from build123d import *

# Parameters (mm, degrees)
SKETCH1_R             = 52.3875
SKETCH1_R_2           = 27.49999999
BOSS_EXTRUDE1_DEPTH   = 11.43
M6_CLEARANCE_HOLE1_D  = 6.6
F_5_0MM_DOWEL_HOLE1_D = 5
CIRPATTERN1_COUNT     = 4
CUT_EXTRUDE1_DEPTH    = 284.979078357
CUT_EXTRUDE2_DEPTH    = 284.979078357


with BuildPart() as part:
    # Sketch1 → Boss-Extrude1 (new body)
    with BuildSketch(Plane(origin=(0, 0, 0), x_dir=(1, 0, 0), z_dir=(0, 1, 0))):
        with BuildLine():
            Line((-207.974881785, -9.956762437), (-62.780706514, -68.14502812))
            ThreePointArc((-62.780706514, -68.14502812), (-33.518744337, -68.231765471), (-12.176603989, -48.212200061))
            Line((-12.176603989, -48.212200061), (1.412558245, -19.284326264))
            ThreePointArc((1.412558245, -19.284326264), (9.075779399, -13.857488875), (17.670000792, -17.640990049))
            Line((17.670000792, -17.640990049), (83.271163186, -105.631794066))
            ThreePointArc((83.271163186, -105.631794066), (87.219797031, -141.651403947), (57.667100455, -162.619048791))
            Line((57.667100455, -162.619048791), (-117.895657849, -177.687193688))
            ThreePointArc((-117.895657849, -177.687193688), (-142.761859432, -174.739029029), (-164.426538493, -162.182702446))
            ThreePointArc((-164.426538493, -162.182702446), (-168.164823601, -160.06920649), (-172.443362527, -159.700770109))
            Line((-172.443362527, -159.700770109), (-204.355245166, -163.82191268))
            ThreePointArc((-204.355245166, -163.82191268), (-214.295764489, -158.206433226), (-211.707233022, -147.086764223))
            Line((-211.707233022, -147.086764223), (-198.151371623, -135.681934472))
            ThreePointArc((-198.151371623, -135.681934472), (-188.283833694, -119.954004575), (-189.430137427, -101.422354045))
            Line((-189.430137427, -101.422354045), (-220.388836369, -22.267635732))
            ThreePointArc((-220.388836369, -22.267635732), (-218.225236723, -12.034965467), (-207.974881785, -9.956762437))
        make_face()
        with Locations(Location((-123.19, -116.001477372, 0), (0, 0, 270))):
            Circle(SKETCH1_R, mode=Mode.SUBTRACT)
        with Locations(Location((54.61, -127, 0), (0, 0, 270))):
            Circle(SKETCH1_R_2, mode=Mode.SUBTRACT)
    extrude(amount=BOSS_EXTRUDE1_DEPTH)

    # M6 Clearance Hole1 (through all)
    with Locations(Plane(origin=(0, 0, 0), x_dir=(-1, 0, 0), z_dir=(0, -1, 0))):
        with Locations((-10.033704867, -23.334197365), (211.518182886, -18.798178744), (205.575185514, -154.375359311)):
            Hole(M6_CLEARANCE_HOLE1_D / 2)

    # Ø5.0mm Dowel Hole1 (through all)
    with Locations(Plane(origin=(0, 0, 0), x_dir=(-1, 0, 0), z_dir=(0, -1, 0))):
        with Locations((123.19, -173.151477372)):
            f_5_0mm_dowel_hole1 = Hole(F_5_0MM_DOWEL_HOLE1_D / 2)

    # CirPattern1: Ø5.0mm Dowel Hole1 ×4 about axis
    cirpattern1_axis = Axis((-123.19, 0, 116.001477372), (0, 1, 0))
    for i in range(1, CIRPATTERN1_COUNT):
        add(f_5_0mm_dowel_hole1.rotate(cirpattern1_axis, i * 360 / CIRPATTERN1_COUNT), mode=Mode.SUBTRACT)

    # Sketch6 → Cut-Extrude1 (cut, through all)
    with BuildSketch(Plane.XZ):
        with BuildLine():
            Line((-14.234653979, 76.580666612), (2.086502597, 40.770912553))
            ThreePointArc((2.086502597, 40.770912553), (11.250375023, 34.121155358), (21.665234735, 38.562610722))
            Line((21.665234735, 38.562610722), (49.771061223, 75.359760223))
            ThreePointArc((49.771061223, 75.359760223), (50.416714446, 82.029052969), (44.724694776, 85.564197365))
            Line((44.724694776, 85.564197365), (-8.456504121, 85.564197365))
            ThreePointArc((-8.456504121, 85.564197365), (-13.797169823, 82.649279585), (-14.234653979, 76.580666612))
        make_face()
        with BuildLine():
            Line((-204.660650751, 36.331409888), (-188.626913597, 77.326218823))
            ThreePointArc((-188.626913597, 77.326218823), (-183.343464985, 81.400582198), (-177.265672517, 78.648182362))
            ThreePointArc((-177.265672517, 78.648182362), (-164.864290964, 65.181201114), (-149.229324423, 55.657458697))
            ThreePointArc((-149.229324423, 55.657458697), (-145.319075006, 49.625624375), (-149.386073966, 43.698348841))
            Line((-149.386073966, 43.698348841), (-194.042740287, 25.801666969))
            ThreePointArc((-194.042740287, 25.801666969), (-202.810079512, 27.579196728), (-204.660650751, 36.331409888))
        make_face()
        with BuildLine():
            Line((-190.985681304, 136.027573744), (-194.692687992, 140.689511725))
            ThreePointArc((-194.692687992, 140.689511725), (-195.773357295, 149.809803058), (-188.096484537, 154.850952212))
            Line((-188.096484537, 154.850952212), (-182.142551509, 155.01295786))
            ThreePointArc((-182.142551509, 155.01295786), (-179.298484939, 153.425933155), (-179.332786017, 150.169219243))
            ThreePointArc((-179.332786017, 150.169219243), (-182.766707481, 143.751485155), (-185.46990532, 136.993390091))
            ThreePointArc((-185.46990532, 136.993390091), (-187.940827525, 134.871620657), (-190.985681304, 136.027573744))
        make_face()
    extrude(amount=-CUT_EXTRUDE1_DEPTH, mode=Mode.SUBTRACT)

    # Sketch7 → Cut-Extrude2 (cut, through all)
    with BuildSketch(Plane.XZ):
        with BuildLine():
            Line((-48.815667356, 114.096477372), (7.572332644, 114.096477372))
            ThreePointArc((7.572332644, 114.096477372), (17.097332644, 104.571477372), (7.572332644, 95.046477372))
            Line((7.572332644, 95.046477372), (-48.815667356, 95.046477372))
            ThreePointArc((-48.815667356, 95.046477372), (-58.340667356, 104.571477372), (-48.815667356, 114.096477372))
        make_face()
        with BuildLine():
            Line((-60.480063265, 159.980626251), (9.143311078, 148.338049571))
            ThreePointArc((9.143311078, 148.338049571), (17.064665217, 138.155302762), (7.572332644, 129.418495204))
            Line((7.572332644, 129.418495204), (-51.525154545, 129.418495204))
            ThreePointArc((-51.525154545, 129.418495204), (-57.140513894, 131.249772802), (-60.59665397, 136.039442314))
            ThreePointArc((-60.59665397, 136.039442314), (-63.415414116, 143.322639291), (-67.078188304, 150.220062883))
            ThreePointArc((-67.078188304, 150.220062883), (-66.914295931, 157.219714512), (-60.480063265, 159.980626251))
        make_face()
    extrude(amount=-CUT_EXTRUDE2_DEPTH, mode=Mode.SUBTRACT)


solid = part.part
The listing builds one solid part. Answer for the finished solid, in the listing's coordinates (mm). A direction names the side the tool comes from. Round coordinates to 2 decimals unless told otherwise and drop trailing zeros. Write each loop counter-clockwise with the first axis right and the second up, starting at its lowest first coordinate (ties: lowest second). Pieces come first, ordered by that corner, then holes. Notation, with made-up numbers: (-40, -4) - (-10, -4) arc R15 ccw to (-10, 23) - close; hole circle Ø7 at (29, 50). An arc over 180 degrees is marked (long way). Use a Markdown table: item, result. Add a question column.
1. The part is cut by section C-C (y = 9.5). Give the number of separate pieces and of enclosed holes in the cut face, and give its area (3 significant figures).
2. Consider line 1 (X direction, y = 3, z = 103); line 2 (X direction, y = 8, z = 16.5); line 3 (X direction, y = 3.75, z = 59). Determine where each line is inside the solid, lowest interval first.
3. The part is cut by section B-B (x = -20.5). Write down the section's boundary in (y, z).
4. The part is cut by section A-A (x = 54.61). Write down the section's boundary in (y, z), and give its area (3 significant figures).
5. A tool of negligible diameter and unlimited length cuts with its end or side. For faces 1 (the face through (50.01, 5.63, 61.02)), 2 (the face through (-188.176, 5.635, 161.732)), 3 (the face through (-26.16, 5.63, 154.24)), from which of +Z, -Z, +X, -X, +Y, -Y can it reach the whole face along a straight path? Write none if from no direction.
6. Flat-ended cylindrical pins translate along their axes: P1, Ø4.5, axis at x = -66.04, z = 116, coming from the +Y side; P2, Ø2, axis at y = 7.5, z = 119.5, coming from the +X side; P3, Ø6, axis at x = -180.34, z = 116, coming from the +Y side; P4, Ø6, axis at x = 49, y = 9.5, coming from the -Z side. Find the tip coordinate at first contact, or state that the pin passes through.
Reported:
| question | item | result |
|---|---|---|
| 1 | separate pieces | 1 |
| 1 | enclosed holes | 14 |
| 1 | area | 16,000 mm^2 |
| 2 | line 1 | -188.86 to -173.94, -72.44 to -58.21, 16.97 to 41.18, 68.04 to 81.31 |
| 2 | line 2 | -220.76 to -213.89, -209.15 to -191.65, 3.4 to 16.67 |
| 2 | line 3 | -206.02 to -195.79, -155.91 to -125.69, -120.69 to -85.6, -19.64 to -6.22, 37.28 to 48.51 |
| 3 | outline | (0, 59.85) - (11.43, 59.85) - (11.43, 95.05) - (0, 95.05) - close; (0, 114.1) - (11.43, 114.1) - (11.43, 129.42) - (0, 129.42) - close; (0, 153.3) - (11.43, 153.3) - (11.43, 169.33) - (0, 169.33) - close |
| 4 | outline | (0, 67.19) - (11.43, 67.19) - (11.43, 99.5) - (0, 99.5) - close; (0, 154.5) - (11.43, 154.5) - (11.43, 162.88) - (0, 162.88) - close |
| 4 | area | 465 mm^2 |
| 5 | face 1 | -Z, +X, +Y, -Y |
| 5 | face 2 | +Z, +Y, -Y |
| 5 | face 3 | +Y, -Y |
| 6 | P1 | through |
| 6 | P2 | x = 89.76 |
| 6 | P3 | y = 11.43 |
| 6 | P4 | z = 55.64 |
